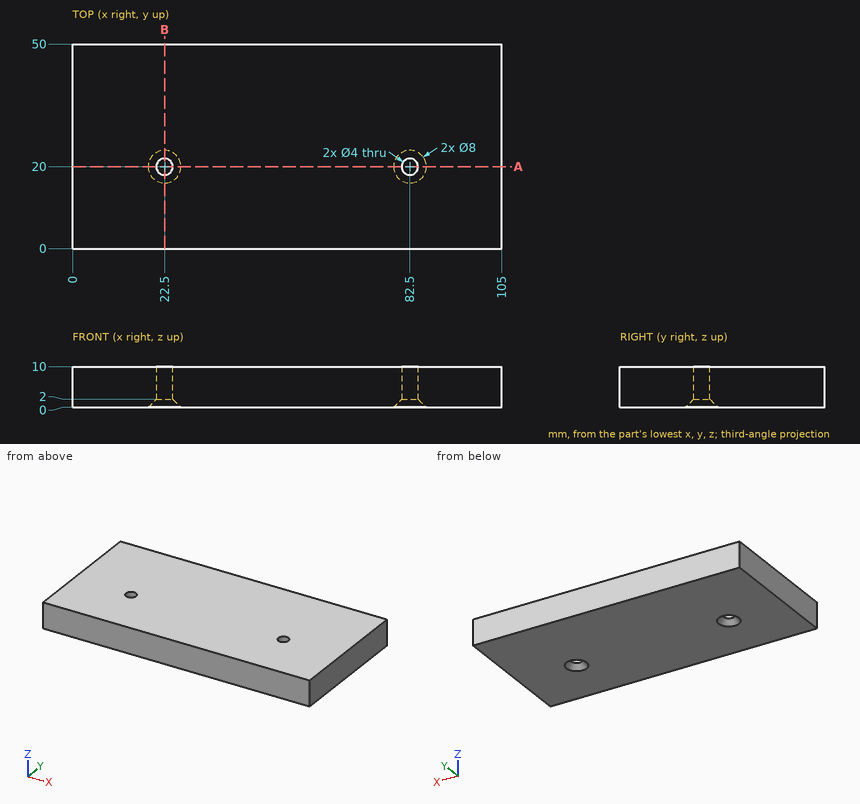
Can you work these out from the drawing? Everything is in mm from the part's minimum corner. Give positions to 0.01 mm unless a question says otherwise; leave off trailing zeros. Loops run counter-clockwise (first coordinate to the right, second up) from the corner with the lowest first, then second, coordinate; pieces in that order, holes last. Notation, with made-up numbers: (40, 42.25) - (81, 42.25) arc R25 cw to (81, 59.25) - close; hole circle Ø4 at (-13.75, 1.25). An arc over 180 degrees is marked (long way). Use one line per item in the form item = value.
1. I'm going to push a flat-ended pin straight in: pin 1 Ø3.5 at (x, y) = (82.5, 20) entering from -Z. Where does the tip first touch, or does it pass through?
Response values:
pin_1 = through
2. I want a section at A-A (y = 20). Please give me the cut outline in (x, z), and give its area (3 significant figures).
Response values:
outline = (0, 0) - (18.5, 0) - (20.5, 2) - (20.5, 10) - (0, 10) - close; (24.5, 2) - (26.5, 0) - (78.5, 0) - (80.5, 2) - (80.5, 10) - (24.5, 10) - close; (84.5, 2) - (86.5, 0) - (105, 0) - (105, 10) - (84.5, 10) - close
area = 962 mm²
3. I want a section at B-B (x = 22.5). Please give me the cut outline in (y, z), and give its area (3 significant figures).
Response values:
outline = (0, 0) - (16, 0) - (18, 2) - (18, 10) - (0, 10) - close; (22, 2) - (24, 0) - (50, 0) - (50, 10) - (22, 10) - close
area = 456 mm²
4. I need wall thicknesses on probe 1 along X at (y, z) = (20, 5.75); probe 2 along Y at (x, z) = (82.5, 7.5); probe 3 along X at (y, z) = (20, 0.5). Which ranges of each line are inside material? Lowest first, please.
Response values:
probe_1 = 0 to 20.5, 24.5 to 80.5, 84.5 to 105
probe_2 = 0 to 18, 22 to 50
probe_3 = 0 to 19, 26 to 79, 86 to 105
